from build123d import *

# Parameters (mm, degrees)
ESQUISSE1_R             = 2.5
BOSS_EXTRU_1_DEPTH      = 20
ESQUISSE2_W             = 10
ESQUISSE2_H             = 20
ENL_V_MAT_EXTRU_1_DEPTH = 10
ENL_V_MAT_EXTRU_2_REACH = 112.675


with BuildPart() as part:
    # Esquisse1 → Boss.-Extru.1 (new body)
    with BuildSketch(Plane.XY):
        Polygon((-102, 0), (-5, -10), (5, -10), (5, 10), (-5, 10), (-92, 10), (-92, 20), (-102, 20), (-102, 10), align=None)
        with Locations((0, 5)):
            Circle(ESQUISSE1_R, mode=Mode.SUBTRACT)
        with Locations((0, -5)):
            Circle(ESQUISSE1_R, mode=Mode.SUBTRACT)
    extrude(amount=BOSS_EXTRU_1_DEPTH)

    # Esquisse2 → Enlèv. mat.-Extru.1 (cut)
    with BuildSketch(Plane.XY.offset(20)):
        Rectangle(ESQUISSE2_W, ESQUISSE2_H)
    extrude(amount=-ENL_V_MAT_EXTRU_1_DEPTH, mode=Mode.SUBTRACT)

    # Enlèv. mat.-Extru.2: up to this face of the body (flat: up to its plane)
    enl_v_mat_extru_2_end = Plane(part.part.faces().sort_by_distance((-5, 0, 15))[0])
    # Esquisse4 → Enlèv. mat.-Extru.2 (cut, up to the picked face)
    with BuildSketch(Plane.ZY.offset(102), mode=Mode.PRIVATE) as enl_v_mat_extru_2_sk1:
        with BuildLine():
            Line((20, 6), (20, -6))
            add(Edge.make_bspline(
                [(20, 6), (16, 0), (20, -6)],
                knots=[0, 0, 0, 1, 1, 1], degree=2))
        make_face()
    enl_v_mat_extru_2_tool1 = split(extrude(enl_v_mat_extru_2_sk1.sketch, amount=-ENL_V_MAT_EXTRU_2_REACH, mode=Mode.PRIVATE), bisect_by=enl_v_mat_extru_2_end, keep=Keep.BOTH, mode=Mode.PRIVATE)
    add(enl_v_mat_extru_2_tool1.solids().sort_by(Axis((-102, 0, 19.2), (1, 0, 0)))[0], mode=Mode.SUBTRACT)


solid = part.part
Can you work these out from the model? Positions are in its coordinate system, mm. A direction names the side the tool comes from. Give positions to 0.01 mm unless a question says otherwise; leave off trailing zeros. Loops run counter-clockwise (first coordinate to the right, second up) from the corner with the lowest first, then second, coordinate; pieces in that order, holes last. Notation, with made-up numbers: (-30.5, 80) - (19.5, 80) arc R21 cw to (19.5, 113) - close; hole circle Ø5 at (-31, -34). An arc over 180 degrees is marked (long way). Answer as a JSON object with one key per item and string values.
Q1. Which directions (+Z, -Z, +X, -X, +Y, -Y) give clear straight access to the entire face, cutting with the end or side of a thin tool? Please do faces 1 (the flat face through (-102, 10, 10)), 2 (the flat face through (-92, 15, 10)), 3 (the flat face through (-5, 0, 15)).
Geometry says:
{"face 1": "+Z, -Z, -X, +Y, -Y", "face 2": "+Z, -Z, +X, +Y", "face 3": "+Z, +X, +Y, -Y"}
Q2. Imagine slicing it at A-A on x = 0. Write out the boundary of the cut face in (y, z).
Geometry says:
{"outline": "(-10, 0) - (-7.5, 0) - (-7.5, 10) - (-10, 10) - close; (-2.5, 0) - (2.5, 0) - (2.5, 10) - (-2.5, 10) - close; (7.5, 0) - (10, 0) - (10, 10) - (7.5, 10) - close"}
Q3. Imagine slicing it at C-C on y = 8.5. Write out the boundary of the cut face in (x, z), plus the area to 3 significant figures.
Geometry says:
{"outline": "(-102, 0) - (5, 0) - (5, 10) - (-5, 10) - (-5, 20) - (-102, 20) - close", "area": "2,040 mm²"}
Q4. If we mould it in two halves opening along Y, with no side actions, what happens to faces 4 (the flat face through (-97, 20, 10)), 5 (the cylindrical face through (-0.33, 7.48, 4.93)), 6 (the flat face through (-65, 8, 20)), 7 (the cylindrical face through (-0.33, -2.52, 4.93))? For each: pulls with the +Y half, pulls with the -Y half, needs draft (parallel to the pull), parting line crosses it, or undercut.
Geometry says:
{"face 4": "pulls with the +Y half", "face 5": "undercut", "face 6": "needs draft", "face 7": "undercut"}
Q5. Imagine slicing it at B-B on z = 2.25. Write out the boundary of the cut face in (x, y), plus the area to 3 significant figures.
Geometry says:
{"outline": "(-102, 0) - (-5, -10) - (5, -10) - (5, 10) - (-92, 10) - (-92, 20) - (-102, 20) - close; hole circle Ø5 at (0, -5); hole circle Ø5 at (0, 5)", "area": "1,720 mm²"}
Q6. Imagine slicing it at D-D on z = 16.25. Write out the boundary of the cut face in (x, y), plus the area to 4 significant figures.
Geometry says:
{"outline": "(-102, 0) - (-5, -10) - (-5, 10) - (-92, 10) - (-92, 20) - (-102, 20) - close", "area": "1,555 mm²"}
Q7. Will these pins go through, and if not, where does the flat tip stop? P1, Ø6.5, axis at x = 0, y = 5, coming from the +Z side; P2, Ø6, axis at x = -65.5, z = 9.5, coming from the -Y side; P3, Ø5, axis at x = -47.5, z = 9, coming from the +Y side.
Geometry says:
{"P1": "z = 10", "P2": "y = -4.07", "P3": "y = 10"}
Q8. If I drill on L1, parallel to Y at x = 0, z = 4; L2, parallel to Z at x = -28, y = -0.5; L3, parallel to X at y = 12.5, z = 11, over which ranges is the centre line in solid material (lowest first)?
Geometry says:
{"L1": "-10 to -7.5, -2.5 to 2.5, 7.5 to 10", "L2": "0 to 18.01", "L3": "-102 to -92"}
